The listing builds one solid part. Answer for the finished solid, in the listing's coordinates (mm). Face numbers are marked on the shaded views. A direction names the side the tool comes from. Give positions to 0.01 mm unless a question says otherwise; leave off trailing zeros. Write each loop counter-clockwise with the first axis right and the second up, starting at its lowest first coordinate (ties: lowest second). Pieces come first, ordered by that corner, then holes. Notation, with made-up numbers: (77.5, 64) -> (118.5, 64) arc R14 ccw to (118.5, 90) -> close; hole circle Ø3 at (-15.5, 0). An arc over 180 degrees is marked (long way). One line per question, with ' | ' between items.
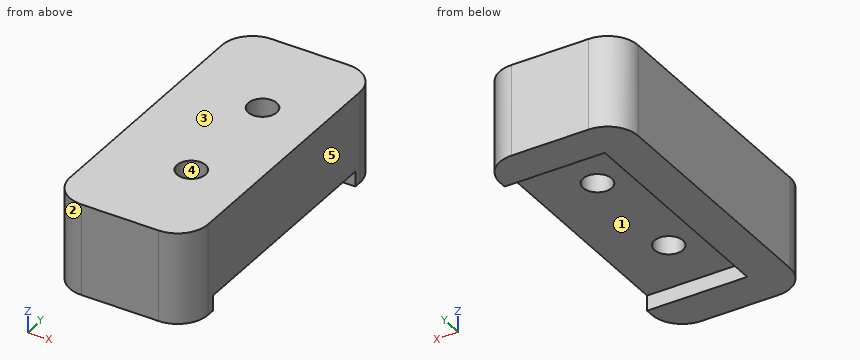
from build123d import *

# Parameters (mm, degrees)
F1_W     = 23.01875
F1_H     = 50.8
F1_R     = 2.38125
F2_DEPTH = 12.7
F4_DEPTH = 2.54
F5_R     = 5.08


with BuildPart() as f2:
    # F1 (on Top) → F2 (new body)
    with BuildSketch(Plane.XY):
        with Locations((-221.059375, 19.05)):
            Rectangle(F1_W, F1_H)
        with Locations((-219.075, 9.525)):
            Circle(F1_R, mode=Mode.SUBTRACT)
        with Locations((-219.075, 28.575)):
            Circle(F1_R, mode=Mode.SUBTRACT)
    extrude(amount=F2_DEPTH)

    # F3 (on face) → F4 (join)
    with BuildSketch(Plane(origin=(0, 0, 0), x_dir=(1, 0, 0), z_dir=(0, 0, -1))):
        Polygon((-209.55, 6.35), (-232.56875, 6.35), (-232.56875, -44.45), (-209.55, -44.45), (-209.55, -38.1), (-226.21875, -38.1), (-226.21875, 0), (-209.55, 0), align=None)
    extrude(amount=F4_DEPTH)

    # F5
    f5_edges = [f2.edges().sort_by_distance(p)[0] for p in [
        (-209.55, -6.35, 5.08),
        (-232.56875, -6.35, 5.08),
        (-232.56875, 44.45, 5.08),
        (-209.55, 44.45, 5.08),
    ]]
    fillet(f5_edges, radius=F5_R)


solid = f2.part
Item 1: Consider line 1 (X direction, y = 9.5, z = 5); line 2 (Y direction, x = -217, z = 5.25); line 3 (Y direction, x = -221.75, z = -1.5). Determine where each line is inside the solid, lowest interval first. Write a range as [from, to].
Answers below:
line 1: [-232.57, -221.46], [-216.69, -209.55] | line 2: [-6.35, 8.36], [10.69, 27.41], [29.74, 44.45] | line 3: [-6.35, 0], [38.1, 44.45]
Item 2: A tool of negligible diameter and unlimited length cuts with its end or side. For the marked faces 1 and 2, from which of +Z, -Z, +X, -X, +Y, -Y can it reach the whole face along a straight path? Write none if from no direction.
Answers below:
face 1: -Z, +X | face 2: +Z, -Z, -X, -Y
Item 3: Find section D-D (z = 10). Count the separate pieces of the cut face and the enclosed holes in it, then the cut area to 3 significant figures.
Answers below:
separate pieces: 1 | enclosed holes: 2 | area: 1,110 mm²
Item 4: Find section C-C (y = 21). Write down the section's boundary in (x, z), then the cut area to 3 significant figures.
Answers below:
outline: (-232.57, -2.54) -> (-226.22, -2.54) -> (-226.22, 0) -> (-209.55, 0) -> (-209.55, 12.7) -> (-232.57, 12.7) -> close | area: 308 mm²
Item 5: Find section B-B (x = -220.25). Write down the section's boundary in (y, z).
Answers below:
outline: (-6.35, -2.54) -> (0, -2.54) -> (0, 0) -> (7.45, 0) -> (7.45, 12.7) -> (-6.35, 12.7) -> close; (11.6, 0) -> (26.5, 0) -> (26.5, 12.7) -> (11.6, 12.7) -> close; (30.65, 0) -> (38.1, 0) -> (38.1, -2.54) -> (44.45, -2.54) -> (44.45, 12.7) -> (30.65, 12.7) -> close
Item 6: Find section A-A (y = 10). Write down the section's boundary in (x, z), then the cut area to 3 significant figures.
Answers below:
outline: (-232.57, -2.54) -> (-226.22, -2.54) -> (-226.22, 0) -> (-221.41, 0) -> (-221.41, 12.7) -> (-232.57, 12.7) -> close; (-216.74, 0) -> (-209.55, 0) -> (-209.55, 12.7) -> (-216.74, 12.7) -> close | area: 249 mm²
Item 7: Determine the mould class of the marked faces 3, 4 and 5 for opening direction X: pulls with the +X half, pulls with the -X half, needs draft (parallel to the pull), parting line crosses it, or undercut.
Answers below:
face 3: needs draft | face 4: undercut | face 5: pulls with the +X half
Item 8: Flat-ended cylindrical pins translate along their axes: pin 1 (6 mm diameter, centred on x = -218, y = 30.5, fed in from -Z); pin 2 (0.8 mm diameter, centred on y = 18, z = -1.5, fed in from +X). Find the tip coordinate at first contact, or state that the pin passes through.
Answers below:
pin 1: z = 0 | pin 2: x = -226.22
